Source: CAD feature listing. Evaluate the final solid. Frame: model axes, mm. A direction names the side the tool comes from. Coordinates: 2 decimals unless noted, no trailing zeros. Order: outer loops, then holes, each group sorted by start corner. A loop starts at its lowest first (then second) coordinate and runs counter-clockwise, first axis right, second up. Notation, with made-up numbers: (32, -15) - (82, -15) arc R30 ccw to (82, 18) - close; hole circle Ø1 at (-21, -2). An arc over 180 degrees is marked (long way). One line per question, with ' | ' between items. Start each with the question number.
(1) Access query for faces 4 (the cylindrical face through (-2.44, -0.07, 0.54)), 5 (the flat face through (6, -3.675, -2)), 6 (the flat face through (-2.1, -4.5, -2.1)). Directions: +Z, -Z, +X, -X, +Y, -Y. A direction counts if a zero-diameter tool reaches every point of the face in a straight line with its end or side. Return the directions, or none.
(2) Section C-C (y = -2.5). Return the cut outline in (x, z), then the cut area to 3 significant figures.
(3) Draft query along Y for faces 1 (the cylindrical face through (-2.703, 4.093, -8.584)), 2 (the flat face through (6, 3.675, 2)), 3 (the flat face through (-2.1, 4.5, 2.1)). Return one class per face: +Y half, -Y half, draft (parallel to the pull), parting line (faces both ways), or undercut.
(4) Contact query for flat-ended pins moving along their axis: P1, Ø5.5, axis at x = -4, z = 1.5, coming from the +Y side; P2, Ø10, axis at x = 5, z = -7, coming from the -Y side; P3, Ø2, axis at x = -2.5, y = -2.5, coming from the -Z side; P4, Ø4, axis at x = 6, z = 1, coming from the +Y side. Output: stop coordinate, or through.
(5) Line query: line 1 along X through (y, z) = (-0.25, 0); line 2 along Y through (x, z) = (0, 7.5) (3 decimals); line 3 along X through (y, z) = (-3, -1.5). Output: solid intervals per line, ascending.
(6) Section D-D (z = 6.75). Return the cut outline in (x, y) (3 decimals), then the cut area to 3 significant figures.
(7) Section A-A (z = 0). Return the cut outline in (x, y) (3 decimals).
(8) Section B-B (x = 0). Return the cut outline in (y, z) (3 decimals), then the cut area to 3 significant figures.
from build123d import *

# Parameters (mm, degrees)
ESBO_O2_R                = 2.8
ESBO_O2_R_2              = 2.5
RESSALTO_EXTRUS_O1_DEPTH = 0.2
RESSALTO_EXTRUS_O2_START = 0.2
ESBO_O4_R                = 2.8
ESBO_O4_R_2              = 2.5
RESSALTO_EXTRUS_O2_DEPTH = 0.2


with BuildPart() as part:
    # Esboço1 → Revolução1 (revolve)
    with BuildSketch(Plane.XY, mode=Mode.PRIVATE) as revolu_o1_sk:
        Polygon((-9, -4.5), (-9, -3.675), (-6.05, -3.675), (-6.05, 3.675), (-9, 3.675), (-9, 4.5), (-2.5, 4.5), (-2.5, -4.5), align=None)
    revolve(revolu_o1_sk.sketch.rotate(Axis((0, 0, 0), (0, 1, 0)), 270), axis=Axis((0, 0, 0), (0, 1, 0)))

    # Esboço2 → Ressalto-extrusão1 (add)
    with BuildSketch(Plane(origin=(0, 4.5, 0), x_dir=(1, 0, 0), z_dir=(0, 1, 0))):
        with Locations(Location((0, 0, 0), (0, 0, 90))):
            Circle(ESBO_O2_R)
        with Locations(Location((0, 0, 0), (0, 0, 90))):
            Circle(ESBO_O2_R_2, mode=Mode.SUBTRACT)
    extrude(amount=RESSALTO_EXTRUS_O1_DEPTH)

    # Esboço4 → Ressalto-extrusão2 (add)
    with BuildSketch(Plane.XZ.offset(4.5).offset(RESSALTO_EXTRUS_O2_START)):
        with Locations(Location((0, 0, 0), (0, 0, 270))):
            Circle(ESBO_O4_R)
        with Locations(Location((0, 0, 0), (0, 0, 270))):
            Circle(ESBO_O4_R_2, mode=Mode.SUBTRACT)
    extrude(amount=-RESSALTO_EXTRUS_O2_DEPTH)


solid = part.part
Response values:
1) face 4: +Y, -Y | face 5: none | face 6: -Y
2) outline: circle Ø12.1 at (0, 0); hole circle Ø5 at (0, 0) | area: 95.4 mm²
3) face 1: draft | face 2: undercut | face 3: +Y half
4) P1: stops at y = 4.7 | P2: stops at y = -4.5 | P3: stops at z = -5.86 | P4: stops at y = 4.5
5) line 1: x = -6.05 to -2.5, 2.5 to 6.05 | line 2: y = -4.5 to -3.675, 3.675 to 4.5 | line 3: x = -5.86 to -2, 2 to 5.86
6) outline: (-5.953, -4.5) - (5.953, -4.5) - (5.953, -3.675) - (-5.953, -3.675) - close; (-5.953, 3.675) - (5.953, 3.675) - (5.953, 4.5) - (-5.953, 4.5) - close | area: 19.6 mm²
7) outline: (-9, -4.5) - (-2.8, -4.5) - (-2.8, -4.7) - (-2.5, -4.7) - (-2.5, 4.7) - (-2.8, 4.7) - (-2.8, 4.5) - (-9, 4.5) - (-9, 3.675) - (-6.05, 3.675) - (-6.05, -3.675) - (-9, -3.675) - close; (2.5, -4.7) - (2.8, -4.7) - (2.8, -4.5) - (9, -4.5) - (9, -3.675) - (6.05, -3.675) - (6.05, 3.675) - (9, 3.675) - (9, 4.5) - (2.8, 4.5) - (2.8, 4.7) - (2.5, 4.7) - close
8) outline: (-4.7, -2.8) - (-4.5, -2.8) - (-4.5, -9) - (-3.675, -9) - (-3.675, -6.05) - (3.675, -6.05) - (3.675, -9) - (4.5, -9) - (4.5, -2.8) - (4.7, -2.8) - (4.7, -2.5) - (-4.7, -2.5) - close; (-4.7, 2.5) - (4.7, 2.5) - (4.7, 2.8) - (4.5, 2.8) - (4.5, 9) - (3.675, 9) - (3.675, 6.05) - (-3.675, 6.05) - (-3.675, 9) - (-4.5, 9) - (-4.5, 2.8) - (-4.7, 2.8) - close | area: 73.9 mm²
